Check sheet for the modelled part. Datum: model origin and axes. Units: mm. Round coordinates to 2 decimals unless told otherwise and drop trailing zeros. Order: outer loops, then holes, each group sorted by start corner. A loop starts at its lowest first (then second) coordinate and runs counter-clockwise, first axis right, second up. Notation, with made-up numbers: (-19, 80) -> (-12, 80) arc R25 ccw to (-12, 105) -> close; hole circle Ø10 at (83, 40.5). An arc over 180 degrees is marked (long way). Answer in a Markdown table with one row per item.
```python
from build123d import *

# Parameters (mm, degrees)
SKETCH1_R                          = 85.725
BOSS_EXTRUDE1_DEPTH                = 6.35
F_3_8_CLEARANCE_HOLE1_D            = 10.0838
F_1_4_0_25_CLEARANCE_DOWEL_HOLE1_D = 6.35
F_10_CLEARANCE_HOLE1_D             = 5.1054
F_10_CLEARANCE_HOLE1_DEPTH         = 6.35


with BuildPart() as part:
    # Sketch1 → Boss-Extrude1 (new body)
    with BuildSketch(Plane(origin=(0, 0, 0), x_dir=(1, 0, 0), z_dir=(0, 1, 0))):
        with Locations(Location((0, 0, 0), (0, 0, 270))):
            Circle(SKETCH1_R)
    extrude(amount=BOSS_EXTRUDE1_DEPTH)

    # 3/8 Clearance Hole1 (through all)
    with Locations(Plane(origin=(0, 6.35, 0), x_dir=(0.9997060077974086, 0, 0.024246607469250614), z_dir=(0, 1, 0))):
        with Locations((-62.211704865, -1.508866383), (62.211704865, 1.508866383)):
            Hole(F_3_8_CLEARANCE_HOLE1_D / 2)

    # 1/4 (0.25) Clearance Dowel Hole1 (through all)
    with Locations(Plane(origin=(43.377433792, 6.35, -259.284531313), x_dir=(0.9888467421616725, 0, -0.14893663255306588), z_dir=(0, 1, 0))):
        with Locations((-81.510599056, -249.932175164)):
            Hole(F_1_4_0_25_CLEARANCE_DOWEL_HOLE1_D / 2)

    # #10 Clearance Hole1
    with Locations(Plane(origin=(43.377433792, 0, -259.284531313), x_dir=(-0.9888467421616725, 0, 0.14893663255306588), z_dir=(0, -1, 0))):
        with Locations((143.046531821, -240.66384852), (19.974666291, -259.200501808), (40.884325078, -256.051162244), (34.264091761, -212.096924555), (115.516639717, -199.858950395), (128.757106351, -287.767425773), (122.136873034, -243.813188084), (47.504558395, -300.005399933)):
            Hole(F_10_CLEARANCE_HOLE1_D / 2, depth=F_10_CLEARANCE_HOLE1_DEPTH)


solid = part.part
```
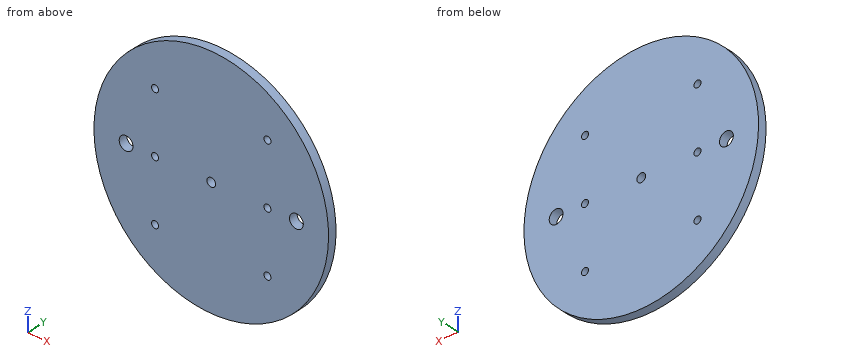
(1) Section check D-D on z = 60.5. Record the boundary of the cut face in (x, y).
Solutions:
| item | result |
|---|---|
| outline | (-60.73, 0) -> (60.73, 0) -> (60.73, 6.35) -> (-60.73, 6.35) -> close |
(2) Section check B-B on x = -62.23. Record the boundary of the cut face in (y, z).
Solutions:
| item | result |
|---|---|
| outline | (0, -58.96) -> (6.35, -58.96) -> (6.35, -5.04) -> (0, -5.04) -> close; (0, 5.04) -> (6.35, 5.04) -> (6.35, 58.96) -> (0, 58.96) -> close |
(3) Section check C-C on z = 38. Record the boundary of the cut face in (x, y), plus the area to 3 significant figures.
Solutions:
| item | result |
|---|---|
| outline | (-76.84, 0) -> (76.84, 0) -> (76.84, 6.35) -> (-76.84, 6.35) -> close |
| area | 976 mm^2 |
(4) Depth check by flat-ended pin: pin 1 Ø2 at (y, z) = (4.5, 15) entering from -X. Enter the tip coordinate at first touch or a pass-through.
Solutions:
| item | result |
|---|---|
| pin 1 | x = -84.57 |
(5) Scan lines: probe 1 along X at (y, z) = (2.5, 0) (3 decimals); probe 2 along X at (y, z) = (2.75, 44.45); probe 3 along Z at (x, y) = (43, 4.25). Record each from-to range of solid material in increasing order. Write a range as from..to.
Solutions:
| item | result |
|---|---|
| probe 1 | -85.725..-67.272, -57.188..-43.637, -38.532..-3.175, 3.175..38.532, 43.637..57.188, 67.272..85.725 |
| probe 2 | -73.3..-43.64, -38.53..38.53, 43.64..73.3 |
| probe 3 | -74.16..-46.14, -42.76..-1.69, 1.69..42.76, 46.14..74.16 |
(6) Section check A-A on y = 4.25. Give the number of separate pieces and of enclosed holes in the cut face, plus the area to 3 significant figures.
Solutions:
| item | result |
|---|---|
| separate pieces | 1 |
| enclosed holes | 9 |
| area | 22,800 mm^2 |
